For this review, take the finished solid that the model builds, in its own axes (mm). A direction names the side the tool comes from. Give positions to 0.01 mm unless a question says otherwise; leave off trailing zeros. Write each loop counter-clockwise with the first axis right and the second up, starting at its lowest first coordinate (ties: lowest second). Pieces come first, ordered by that corner, then holes.
1) We need section A-A on z = 0. Give the boundary of the cut face in (x, y).
2) Draft analysis for pull direction X (two halves, no side actions). For faces 1 (the face through (-7, 0, 230)), 2 (the face through (5.5, -5, -3)), 3 (the face through (7.5, 6, -3)), state which applies: pulls with the +X half, pulls with the -X half, needs draft (parallel to the pull), parting line crosses it, or undercut.
3) We need section B-B on y = 0. Give the boundary of the cut face in (x, z).
4) We need section C-C on z = 165. Give the boundary of the cut face in (x, y), and give its area (3 significant figures).
5) Wall thickness on line 1 along Z through (x, y) = (0, 14); line 2 along X through (y, z) = (5.25, 34.5); line 3 along X through (y, z) = (-13.7, 220): over which ranges is each line inside the solid? List them lowest first.
6) For P1, Ø8, axis at y = 0, z = 0, coming from the -X side; P2, Ø8, axis at x = 0, z = -220, coming from the -Y side, all flat-tipped, find the tip position at first contact; note any pin that passes through.
7) Machinability: for faces 4 (the face through (6.51, -4.88, 1.08)), 5 (the face through (-5.5, 5, -3)), which of the approach directions +Z, -Z, +X, -X, +Y, -Y give a long, thin tool a straight path to every point of the face, cutting with its end or side? Answer none if there is none.
8) We need section D-D on x = 0. Give the boundary of the cut face in (y, z).
Autodesk Inventor part; units mm, degrees
ref_plane "YZ Plane" through (0, 0, 0) normal (1, 0, 0) x (0, 1, 0)
ref_plane "XZ Plane" through (0, 0, 0) normal (0, 1, 0) x (-1, 0, 0)
ref_plane "XY Plane" through (0, 0, 0) normal (0, 0, 1) x (1, 0, 0)
sketch "Sketch1" plane through (0, 0, 0) normal (0, 0, 1) x (1, 0, 0)
  line L0 (-7.5, 15) -> (7.5, 15)
  line L1 (7.5, 15) -> (7.5, -15)
  line L2 (7.5, -15) -> (-7.5, -15)
  line L3 (-7.5, -15) -> (-7.5, 15)
  line L4 (-7.5, 15) -> (7.5, -15) construction
  line L5 (7.5, 15) -> (-7.5, -15) construction
  line L6 (-5.5, 13) -> (5.5, 13)
  line L7 (5.5, 13) -> (5.5, -13)
  line L8 (5.5, -13) -> (-5.5, -13)
  line L9 (-5.5, -13) -> (-5.5, 13)
  point P0 (0, 0)
  dimension "d0" = 15
  dimension "d1" = 30
  dimension "d2" = 2
extrude "Extrusion1" add sketch "Sketch1" along normal mid plane 460
sketch "Sketch2" plane through (-7.5, 15, -230) normal (0, 1, 0) x (1, 0, 0)
  circle A0 centre (7.5, -10) radius 3
  circle A1 centre (7.5, -450) radius 3
  line L0 (15, -460) -> (0, -460)
  line L1 (0, 0) -> (15, 0)
  line L2 (7.5, -450) -> (7.5, -10) construction
  line L3 (0, 0) -> (0, -460) construction
  point P0 (7.5, -230)
  point P1 (7.5, -460)
  point P2 (7.5, 0)
  point P3 (7.5, -230)
  point P4 (0, -230)
  dimension "d5" = 6
  dimension "d6" = 6
  dimension "d7" = 440
extrude "Extrusion2" cut sketch "Sketch2" against normal through all
sketch "Sketch3" plane through (7.5, -15, -230) normal (1, 0, 0) x (0, 0, -1)
  line L0 (0, 30) -> (0, 0)
  line L1 (0, 30) -> (-460, 30)
  line L2 (-460, 0) -> (-460, 30)
  line L3 (0, 0) -> (-460, 0)
  circle A0 centre (-230, 15) radius 5
  point P0 (-230, 30)
  point P1 (0, 15)
  dimension "d10" = 10
extrude "Extrusion3" cut sketch "Sketch3" against normal through all contours A0
fillet "Fillet1" radius 1 8 edges at (7.5, 15, 0) (-7.5, 15, 0) (7.5, -15, 0) (-7.5, -15, 0) (-5.5, 13, 0) (5.5, 13, 0) (5.5, -13, 0) (-5.5, -13, 0)
properties part number "balk" material "Stainless Steel"
Results list:
1. outline: (-7.5, -14) arc R1 ccw to (-6.5, -15) - (6.5, -15) arc R1 ccw to (7.5, -14) - (7.5, -5) - (5.5, -5) - (5.5, -12) arc R1 cw to (4.5, -13) - (-4.5, -13) arc R1 cw to (-5.5, -12) - (-5.5, -5) - (-7.5, -5) - close; (-7.5, 5) - (-5.5, 5) - (-5.5, 12) arc R1 cw to (-4.5, 13) - (4.5, 13) arc R1 cw to (5.5, 12) - (5.5, 5) - (7.5, 5) - (7.5, 14) arc R1 ccw to (6.5, 15) - (-6.5, 15) arc R1 ccw to (-7.5, 14) - close
2. face 1: needs draft
2. face 2: undercut
2. face 3: pulls with the +X half
3. outline: (-7.5, -230) - (-5.5, -230) - (-5.5, -5) - (-7.5, -5) - close; (-7.5, 5) - (-5.5, 5) - (-5.5, 230) - (-7.5, 230) - close; (5.5, -230) - (7.5, -230) - (7.5, -5) - (5.5, -5) - close; (5.5, 5) - (7.5, 5) - (7.5, 230) - (5.5, 230) - close
4. outline: (-7.5, -14) arc R1 ccw to (-6.5, -15) - (6.5, -15) arc R1 ccw to (7.5, -14) - (7.5, 14) arc R1 ccw to (6.5, 15) - (-6.5, 15) arc R1 ccw to (-7.5, 14) - close; hole (-5.5, -12) arc R1 ccw to (-4.5, -13) - (4.5, -13) arc R1 ccw to (5.5, -12) - (5.5, 12) arc R1 ccw to (4.5, 13) - (-4.5, 13) arc R1 ccw to (-5.5, 12) - close
4. area: 164 mm2
5. line 1: z = -230 to -223, -217 to 217, 223 to 230
5. line 2: x = -7.5 to -5.5, 5.5 to 7.5
5. line 3: x = -7.5 to -3, 3 to 7.5
6. P1: passes through
6. P2: stops at y = -15
7. face 4: +X, -X
7. face 5: +Z, -Z
8. outline: (-15, -230) - (-13, -230) - (-13, -223) - (-15, -223) - close; (-15, -217) - (-13, -217) - (-13, 217) - (-15, 217) - close; (-15, 223) - (-13, 223) - (-13, 230) - (-15, 230) - close; (13, -230) - (15, -230) - (15, -223) - (13, -223) - close; (13, -217) - (15, -217) - (15, 217) - (13, 217) - close; (13, 223) - (15, 223) - (15, 230) - (13, 230) - close
